from build123d import *

# Parameters (mm, degrees)
SKETCH1_R           = 12.62515314
BOSS_EXTRUDE1_DEPTH = 127.254
SKETCH2_W           = 21.600890372
SKETCH2_H           = 6.08719661
CUT_EXTRUDE1_DEPTH  = 155.702
CUT_EXTRUDE2_DEPTH  = 141.081655767
SKETCH4_W           = 5.08
SKETCH4_H           = 13.653478909
BOSS_EXTRUDE2_DEPTH = 12.755190121
CUT_EXTRUDE3_REACH  = 132.958
SKETCH15_R          = 3.895516075


with BuildPart() as part:
    # Sketch1 → Boss-Extrude1 (new body)
    with BuildSketch(Plane(origin=(0, 0, 0), x_dir=(1, 0, 0), z_dir=(0, 1, 0))):
        with Locations(Location((0, 0, 0), (0, 0, 270))):
            Circle(SKETCH1_R)
    extrude(amount=-BOSS_EXTRUDE1_DEPTH)

    # Sketch2 → Cut-Extrude1 (cut)
    with BuildSketch(Plane(origin=(0, -127.254, 0), x_dir=(-1, 0, 0), z_dir=(0, -1, 0))):
        with Locations((0, -9.581554835)):
            Rectangle(SKETCH2_W, SKETCH2_H)
    extrude(amount=-CUT_EXTRUDE1_DEPTH, mode=Mode.SUBTRACT)

    # Sketch3 → Cut-Extrude2 (cut)
    with BuildSketch(Plane(origin=(0, -127.254, 0), x_dir=(-1, 0, 0), z_dir=(0, -1, 0))):
        with BuildLine():
            Line((3.126169088, 0), (-3.091625783, 0))
            ThreePointArc((-3.091625783, 0), (0.017271652, 3.108897435), (3.126169088, 0))
        make_face()
    extrude(amount=-CUT_EXTRUDE2_DEPTH, mode=Mode.SUBTRACT)

    # Sketch4 → Boss-Extrude2 (add)
    with BuildSketch(Plane.XZ.offset(127.254)):
        with Locations((-8.260445186, 13.364695985)):
            Rectangle(SKETCH4_W, SKETCH4_H)
    boss_extrude2 = extrude(amount=-BOSS_EXTRUDE2_DEPTH)

    # Sketch15 → Cut-Extrude3 (cut, up to next)
    with BuildSketch(Plane.ZY.offset(10.800445186), mode=Mode.PRIVATE) as cut_extrude3_sk1:
        with Locations((15.440577286, -120.904)):
            Circle(SKETCH15_R)
    cut_extrude3_tool1 = extrude(cut_extrude3_sk1.sketch, amount=-CUT_EXTRUDE3_REACH, mode=Mode.PRIVATE) & part.part
    cut_extrude3 = cut_extrude3_tool1.solids().sort_by_distance((-10.800445, -120.904, 15.440577))[0]
    add(cut_extrude3, mode=Mode.SUBTRACT)

    # Mirror2: Boss-Extrude2, Cut-Extrude3 across plane
    add(boss_extrude2.mirror(Plane(origin=(0, 0, 0), x_dir=(0, 0, 1), z_dir=(1, 0, 0))))
    add(cut_extrude3.mirror(Plane(origin=(0, 0, 0), x_dir=(0, 0, 1), z_dir=(1, 0, 0))), mode=Mode.SUBTRACT)


solid = part.part
Read the model definition and answer for the solid it produces. Units are mm, in the model's axes. A direction names the side the tool comes from. Round coordinates to 2 decimals unless told otherwise and drop trailing zeros. Loops run counter-clockwise (first coordinate to the right, second up) from the corner with the lowest first, then second, coordinate; pieces in that order, holes last.
Q1. Consider probe 1 along X at (y, z) = (-115, 17.5); probe 2 along Y at (x, z) = (-7, 15.5); probe 3 along X at (y, z) = (-26, 6.5). Determine where each line is inside the solid, lowest interval first.
Q2. Section D-D on z = -5 is taken. Write down the section's boundary in (x, y).
Q3. Which of the six approach directions +Z, -Z, +X, -X, +Y, -Y give full straight-line access (tool end or side, diameter ignored) to faces 1 (the face through (-10.8, -121, 10)), 2 (the face through (10.8, -121, 10)), 3 (the face through (-8, -114.499, 13)), 4 (the face through (-5.72, -121, 10))?
Q4. Section C-C on x = 9.5 is taken. Write down the section's boundary in (y, z), and give its area (3 significant figures).
Q5. Determine the mould class of faces 5 (the face through (0, -65, 6.538)), 6 (the face through (0, -65, 0)), 7 (the face through (5.72, -121, 10)) for opening direction Z: released by +Z, released by -Z, zero draft, split by the parting line, or undercut.
Q6. Each of these flat-tipped pins is pushed along its axis until it touches: pin 1 (14 mm diameter, centred on y = -121, z = 12.5, fed in from -X); pin 2 (7 mm diameter, centred on x = -1, y = -53.5, fed in from -Z); pin 3 (10 mm diameter, centred on y = -120.9, z = 15.44, fed in from +X); pin 4 (10 mm diameter, centred on y = -80.5, z = -9, fed in from +X). Where does it stop, or does it pass through?
Q7. Section B-B on y = -66 is taken. Write down the section's boundary in (x, z).
Q8. Section A-A on x = 0 is taken. Write down the section's boundary in (y, z).
Output:
1. probe 1: x = -10.8 to -5.72, 5.72 to 10.8
1. probe 2: y = -127.25 to -124.8, -117.01 to -114.5
1. probe 3: x = -10.82 to 10.82
2. outline: (-11.59, -127.25) - (11.59, -127.25) - (11.59, 0) - (-11.59, 0) - close
3. face 1: +Z, -X, +Y, -Y
3. face 2: +Z, +X, +Y, -Y
3. face 3: +Z, +X, -X, +Y
3. face 4: +Z, +Y, -Y
4. outline: (-127.25, -8.32) - (0, -8.32) - (0, 6.54) - (-114.5, 6.54) - (-114.5, 20.19) - (-127.25, 20.19) - close; hole circle Ø7.79 at (-120.9, 15.44)
4. area: 2,020 mm2
5. face 5: released by +Z
5. face 6: undercut
5. face 7: zero draft
6. pin 1: stops at x = -11.36
6. pin 2: stops at z = -12.63
6. pin 3: stops at x = 10.8
6. pin 4: stops at x = 11.97
7. outline: (-10.8, 6.54) arc R12.63 ccw (long way) to (10.8, 6.54) - close; hole (-3.13, 0) arc R3.11 ccw to (3.09, 0) - close
8. outline: (-127.25, -12.63) - (0, -12.63) - (0, -3.11) - (-127.25, -3.11) - close; (-127.25, 0) - (0, 0) - (0, 6.54) - (-127.25, 6.54) - close
